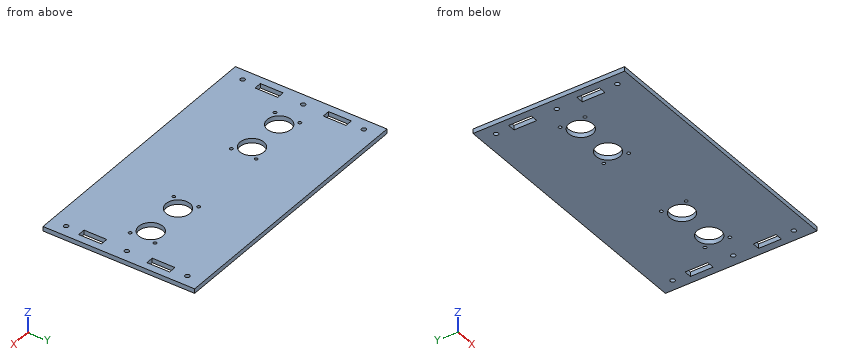
from build123d import *

# Parameters (mm, degrees)
SCHIZZO1_W                   = 180.34
SCHIZZO1_H                   = 100
ESTRUSIONE_ESTRUSIONE1_DEPTH = 3
SCHIZZO2_R                   = 1.5
SCHIZZO2_W                   = 5
SCHIZZO2_H                   = 15
TAGLIO_ESTRUSIONE1_DEPTH     = 4
SCHIZZO3_R                   = 7.94
SCHIZZO3_R_2                 = 1.05
TAGLIO_ESTRUSIONE2_DEPTH     = 4


with BuildPart() as part:
    # Schizzo1 → Estrusione-Estrusione1 (new body)
    with BuildSketch(Plane.XY):
        Rectangle(SCHIZZO1_W, SCHIZZO1_H)
    extrude(amount=ESTRUSIONE_ESTRUSIONE1_DEPTH)

    # Schizzo2 → Taglio-Estrusione1 (cut, through all)
    with BuildSketch(Plane.XY):
        with Locations((-82.67, 0)):
            Circle(SCHIZZO2_R)
        with Locations((82.67, 0)):
            Circle(SCHIZZO2_R)
        with Locations((-82.67, 40)):
            Circle(SCHIZZO2_R)
        with Locations((-82.67, -40)):
            Circle(SCHIZZO2_R)
        with Locations((82.67, -40)):
            Circle(SCHIZZO2_R)
        with Locations((82.67, 40)):
            Circle(SCHIZZO2_R)
        with Locations((-82.67, 22.5)):
            Rectangle(SCHIZZO2_W, SCHIZZO2_H)
        with Locations((-82.67, -22.5)):
            Rectangle(SCHIZZO2_W, SCHIZZO2_H)
        with Locations((82.67, 22.5)):
            Rectangle(SCHIZZO2_W, SCHIZZO2_H)
        with Locations((82.67, -22.5)):
            Rectangle(SCHIZZO2_W, SCHIZZO2_H)
    extrude(amount=TAGLIO_ESTRUSIONE1_DEPTH, mode=Mode.SUBTRACT)

    # Schizzo3 → Taglio-Estrusione2 (cut, through all)
    with BuildSketch(Plane.XY):
        with Locations((-60.17, 0)):
            Circle(SCHIZZO3_R)
        with Locations((-34.67, 0)):
            Circle(SCHIZZO3_R)
        with Locations((60.17, 0)):
            Circle(SCHIZZO3_R)
        with Locations((34.67, 0)):
            Circle(SCHIZZO3_R)
        with Locations((-26.97, -8.2)):
            Circle(SCHIZZO3_R_2)
        with Locations((-26.97, 8.2)):
            Circle(SCHIZZO3_R_2)
        with Locations((-67.87, -8.2)):
            Circle(SCHIZZO3_R_2)
        with Locations((-67.87, 8.2)):
            Circle(SCHIZZO3_R_2)
        with Locations((26.97, 8.2)):
            Circle(SCHIZZO3_R_2)
        with Locations((26.97, -8.2)):
            Circle(SCHIZZO3_R_2)
        with Locations((67.87, -8.2)):
            Circle(SCHIZZO3_R_2)
        with Locations((67.87, 8.2)):
            Circle(SCHIZZO3_R_2)
    extrude(amount=TAGLIO_ESTRUSIONE2_DEPTH, mode=Mode.SUBTRACT)


solid = part.part
Here's how the part is built. I have some questions about the finished solid (model axes, mm). Round coordinates to 2 decimals unless told otherwise and drop trailing zeros. Write each loop counter-clockwise with the first axis right and the second up, starting at its lowest first coordinate (ties: lowest second). Pieces come first, ordered by that corner, then holes. Notation, with made-up numbers: (27.5, 9) -> (66.5, 9) arc R16 cw to (66.5, 35) -> close; hole circle Ø6 at (52, 11.5). An arc over 180 degrees is marked (long way). One line per item, written item: value.
1) Suppose I cut it at D-D on z = 0.9. Give the number of separate pieces and of enclosed holes in the cut face, plus the area to 3 significant figures.
Filled sheet:
separate pieces: 1
enclosed holes: 22
area: 16,900 mm2
2) I'm going to push a flat-ended pin straight in: pin 1 Ø1.9 at (x, y) = (-67.87, -8.2) entering from -Z. Where does the tip first touch, or does it pass through?
Filled sheet:
pin 1: passes through
3) If I drill on line 1 (X direction, y = 8.2, z = 1.1); line 2 (Y direction, x = 82.67, z = 0.7); line 3 (X direction, y = 40, z = 1.85), over which ranges is the centre line in solid material (lowest first)? Write a range as [from, to].
Filled sheet:
line 1: x = [-90.17, -68.92], [-66.82, -28.02], [-25.92, 25.92], [28.02, 66.82], [68.92, 90.17]
line 2: y = [-50, -41.5], [-38.5, -30], [-15, -1.5], [1.5, 15], [30, 38.5], [41.5, 50]
line 3: x = [-90.17, -84.17], [-81.17, 81.17], [84.17, 90.17]
4) Suppose I cut it at B-B on x = 31. List the corners of the cut face in (y, z) for me, plus the area to 3 significant figures.
Filled sheet:
outline: (-50, 0) -> (-7.04, 0) -> (-7.04, 3) -> (-50, 3) -> close; (7.04, 0) -> (50, 0) -> (50, 3) -> (7.04, 3) -> close
area: 258 mm2
5) Suppose I cut it at C-C on y = -3.5. List the corners of the cut face in (x, z) for me.
Filled sheet:
outline: (-90.17, 0) -> (-67.3, 0) -> (-67.3, 3) -> (-90.17, 3) -> close; (-53.04, 0) -> (-41.8, 0) -> (-41.8, 3) -> (-53.04, 3) -> close; (-27.54, 0) -> (27.54, 0) -> (27.54, 3) -> (-27.54, 3) -> close; (41.8, 0) -> (53.04, 0) -> (53.04, 3) -> (41.8, 3) -> close; (67.3, 0) -> (90.17, 0) -> (90.17, 3) -> (67.3, 3) -> close
6) Suppose I cut it at A-A on y = -24.5. List the corners of the cut face in (x, z) for me.
Filled sheet:
outline: (-90.17, 0) -> (-85.17, 0) -> (-85.17, 3) -> (-90.17, 3) -> close; (-80.17, 0) -> (80.17, 0) -> (80.17, 3) -> (-80.17, 3) -> close; (85.17, 0) -> (90.17, 0) -> (90.17, 3) -> (85.17, 3) -> close
